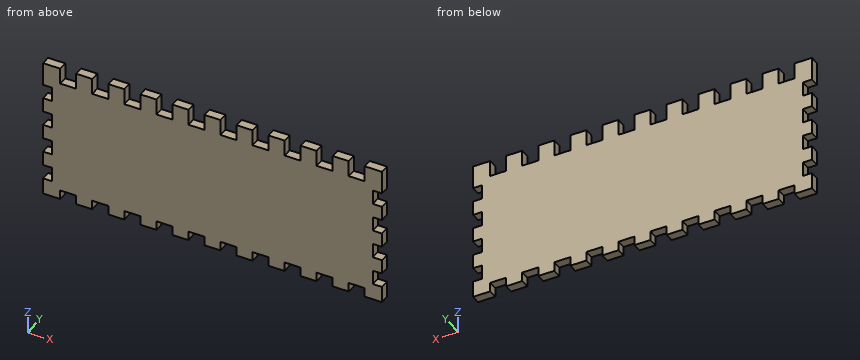
```python
from build123d import *

# Parameters (mm, degrees)
SCHIZZO1_W                   = 140
SCHIZZO1_H                   = 50
ESTRUSIONE_ESTRUSIONE1_DEPTH = 4
ESTRUSIONE_ESTRUSIONE2_DEPTH = 4
SCHIZZO3_W                   = 4
SCHIZZO3_H                   = 6.25
ESTRUSIONE_ESTRUSIONE3_DEPTH = 4
RIPETIZIONE_A_L1_COUNT       = 3
RIPETIZIONE_A_L1_PITCH       = 12.5
SCHIZZO4_W                   = 7
SCHIZZO4_H                   = 4
SCHIZZO4_H_2                 = 7
ESTRUSIONE_ESTRUSIONE4_DEPTH = 4
RIPETIZIONE_A_L2_COUNT       = 9
RIPETIZIONE_A_L2_PITCH       = 14


with BuildPart() as part:
    # Schizzo1 → Estrusione-Estrusione1 (new body)
    with BuildSketch(Plane(origin=(0, 0, 0), x_dir=(1, 0, 0), z_dir=(0, 1, 0))):
        with Locations((70, 25)):
            Rectangle(SCHIZZO1_W, SCHIZZO1_H)
    extrude(amount=ESTRUSIONE_ESTRUSIONE1_DEPTH)

    # Schizzo2 → Estrusione-Estrusione2 (add)
    with BuildSketch(Plane(origin=(0, 4, 0), x_dir=(1, 0, 0), z_dir=(0, 1, 0))):
        Polygon((0, 3.125), (0, 0), (3.5, 0), (3.5, -7), (-4, -7), (-4, 3.125), align=None)
        Polygon((0, 46.875), (-4, 46.875), (-4, 54), (3.5, 54), (3.5, 50), (0, 50), align=None)
        Polygon((136.5, 50), (136.5, 54), (144, 54), (144, 46.875), (140, 46.875), (140, 50), align=None)
        Polygon((140, 3.125), (144, 3.125), (144, -7), (136.5, -7), (136.5, 0), (140, 0), align=None)
    extrude(amount=-ESTRUSIONE_ESTRUSIONE2_DEPTH)

    # Schizzo3 → Estrusione-Estrusione3 (add)
    with BuildSketch(Plane(origin=(0, 4, 0), x_dir=(1, 0, 0), z_dir=(0, 1, 0))):
        with Locations((-2, 37.5)):
            Rectangle(SCHIZZO3_W, SCHIZZO3_H)
        with Locations((142, 37.5)):
            Rectangle(SCHIZZO3_W, SCHIZZO3_H)
    estrusione_estrusione3 = extrude(amount=-ESTRUSIONE_ESTRUSIONE3_DEPTH)

    # Ripetizione a L1: Estrusione-Estrusione3 ×3
    with Locations(*[(0, 0, i * RIPETIZIONE_A_L1_PITCH) for i in range(1, RIPETIZIONE_A_L1_COUNT)]):
        add(estrusione_estrusione3)

    # Schizzo4 → Estrusione-Estrusione4 (add)
    with BuildSketch(Plane(origin=(0, 4, 0), x_dir=(1, 0, 0), z_dir=(0, 1, 0))):
        with Locations((14, 52)):
            Rectangle(SCHIZZO4_W, SCHIZZO4_H)
        with Locations((14, -3.5)):
            Rectangle(SCHIZZO4_W, SCHIZZO4_H_2)
    estrusione_estrusione4 = extrude(amount=-ESTRUSIONE_ESTRUSIONE4_DEPTH)

    # Ripetizione a L2: Estrusione-Estrusione4 ×9
    with Locations(*[(i * RIPETIZIONE_A_L2_PITCH, 0, 0) for i in range(1, RIPETIZIONE_A_L2_COUNT)]):
        add(estrusione_estrusione4)


solid = part.part
```
Work out the finished part from the listing and answer in its coordinate system (mm). Give positions to 0.01 mm unless a question says otherwise; leave off trailing zeros. Loops run counter-clockwise (first coordinate to the right, second up) from the corner with the lowest first, then second, coordinate; pieces in that order, holes last. Notation, with made-up numbers: M -39.5,20.25 L -18.5,20.25 A31 ccw -18.5,58.25 Z; hole C 65,-32 d6. An arc over 180 degrees is marked long. One line per item, written item: value. Start each with the question number.
1. Find section B-B (x = 118.5). Give the vertices of the cut face in (y, z).
2. This flat-tipped pin is pushed along its axis until it touches: P1, Ø1.2, axis at y = 2.5, z = -44.5, coming from the +X side. Where does it stop, or does it pass through?
3. Find section A-A (z = -32). Give the vertices of the cut face in (x, y).
4. Find the intervals of material crossed by probe 1 along Z at (x, y) = (78, 1.6); probe 2 along X at (y, z) = (1.3, -5.5), in increasing order.
Reported:
1. outline: M 0,-50 L 4,-50 L 4,0 L 0,0 Z
2. P1: stops at x = 140
3. outline: M 0,0 L 140,0 L 140,4 L 0,4 Z
4. probe 1: z = -50 to 0
4. probe 2: x = 0 to 140
